Part print with two shaded views. Sizes in mm from the minimum x, y, z corner. Round coordinates to 2 decimals unless told otherwise and drop trailing zeros. Order: outer loops, then holes, each group sorted by start corner. A loop starts at its lowest first (then second) coordinate and runs counter-clockwise, first axis right, second up. Notation, with made-up numbers: (-2.5, 59.5) - (22.5, 59.5) arc R5 ccw to (22.5, 65.5) - close; hole circle Ø1 at (83, 65). An arc over 180 degrees is marked (long way). Use one line per item in the form item = value.
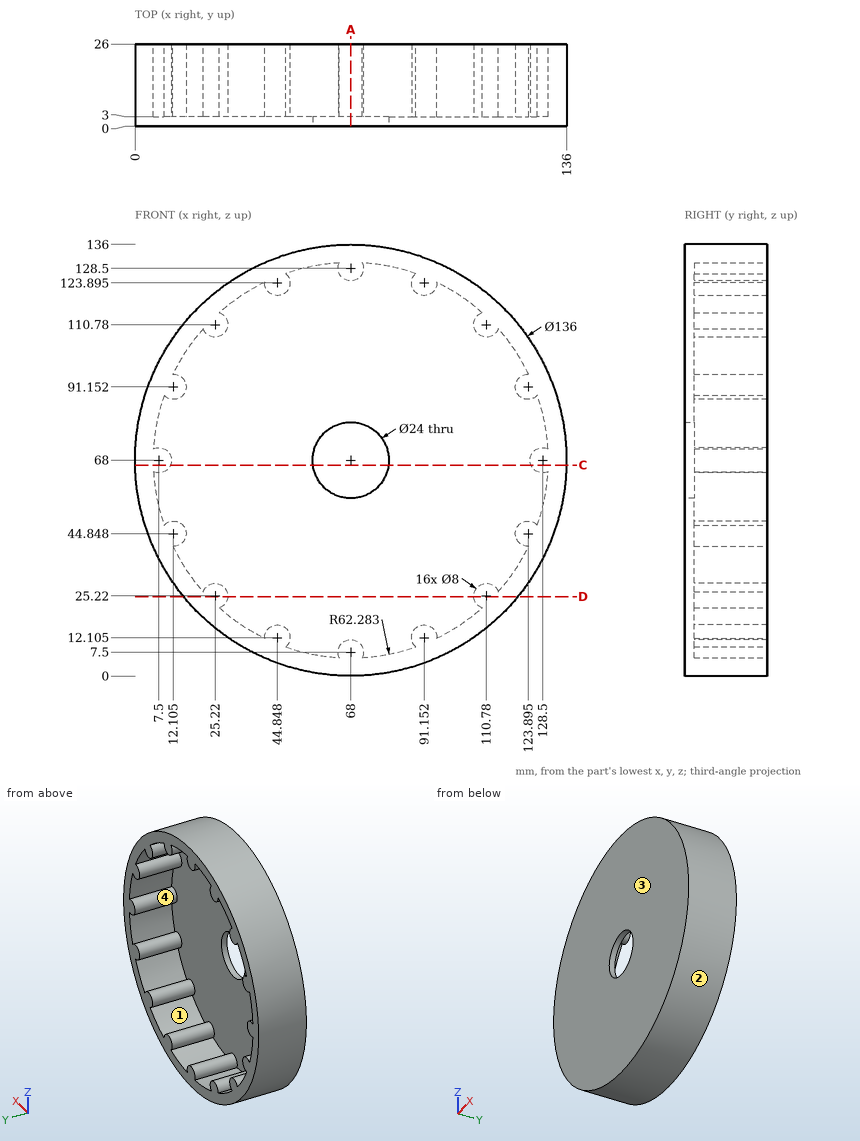
(1) Pull direction Z, two halves, no side cores. Call the marked faces 1, 2, 3 and 4: released by +Z, released by -Z, zero draft, split by the parting line, or undercut.
Report:
face_1 = undercut
face_2 = split by the parting line
face_3 = zero draft
face_4 = undercut
(2) Slice it at D-D on z = 25. Give the cut face in (x, y), then the cut area to 3 significant figures.
Report:
outline = (15.32, 0) - (120.68, 0) - (120.68, 26) - (106.79, 26) - (106.79, 3) - (29.21, 3) - (29.21, 26) - (15.32, 26) - close
area = 955 mm2
(3) Pin check, flat tips, straight feed: pin 1 (6 mm diameter, centred on x = 79, y = 10.5, fed in from +Z); pin 2 (4 mm diameter, centred on y = 18, z = 78.5, fed in from -X); pin 3 (6 mm diameter, centred on y = 3, z = 67, fed in from -X). Stop position of each tip, or through.
Report:
pin_1 = 135.53
pin_2 = 0.53
pin_3 = 0
(4) Probe probe 1 along X at (y, z) = (1.55, 68); probe 2 along Y at (x, z) = (108.5, 97.5); probe 3 along X at (y, z) = (20.25, 48) (1 decimal). List the from-to ranges inside material, lowest first. Write a range as [from, to].
Report:
probe_1 = [0, 56], [80, 136]
probe_2 = [0, 3]
probe_3 = [3, 9], [9.6, 14.6], [121.4, 126.4], [127, 133]
(5) Slice it at A-A on x = 68. Give the cut face in (y, z), then the cut area to 3 significant figures.
Report:
outline = (0, 0) - (26, 0) - (26, 11.5) - (3, 11.5) - (3, 56) - (0, 56) - close; (0, 80) - (3, 80) - (3, 124.5) - (26, 124.5) - (26, 136) - (0, 136) - close
area = 865 mm2
(6) Slice it at C-C on z = 66.5. Give the cut face in (x, y).
Report:
outline = (0.02, 0) - (56.09, 0) - (56.09, 3) - (11.21, 3) - (11.21, 26) - (0.02, 26) - close; (79.91, 0) - (135.98, 0) - (135.98, 26) - (124.79, 26) - (124.79, 3) - (79.91, 3) - close
